Work out the finished part from the listing and answer in its coordinate system (mm). Face numbers are marked on the shaded views. A direction names the side the tool comes from. Give positions to 0.01 mm unless a question says otherwise; leave off trailing zeros. Order: outer loops, then holes, each group sorted by start corner. A loop starts at its lowest first (then second) coordinate and runs counter-clockwise, first axis right, second up.
```python
from build123d import *

# Parameters (mm, degrees)
SKETCH1_R                = 6.5
SKETCH1_R_2              = 5.5
BOSS_EXTRUDE1_DEPTH      = 7.5
BOSS_EXTRUDE2_START      = -2.5
BOSS_EXTRUDE2_DEPTH      = 2.5
M3_CLEARANCE_HOLE1_D     = 3.2
M3_CLEARANCE_HOLE1_DEPTH = 5
M3_CLEARANCE_HOLE1_TIP   = 0.96137699


with BuildPart() as part:
    # Sketch1 → Boss-Extrude1 (new body)
    with BuildSketch(Plane(origin=(0, 0, 0), x_dir=(1, 0, 0), z_dir=(0, 1, 0))):
        with Locations(Location((0, 0, 0), (0, 0, 270))):
            Circle(SKETCH1_R)
        with Locations(Location((0, 0, 0), (0, 0, 270))):
            Circle(SKETCH1_R_2, mode=Mode.SUBTRACT)
    extrude(amount=BOSS_EXTRUDE1_DEPTH)

    # Sketch2 → Boss-Extrude2 (add)
    with BuildSketch(Plane(origin=(0, 7.5, 0), x_dir=(1, 0, 0), z_dir=(0, 1, 0)).offset(BOSS_EXTRUDE2_START)):
        with BuildLine():
            Line((-13.75, 2.5), (-6, 2.5))
            ThreePointArc((-6, 2.5), (-6.5, 0), (-6, -2.5))
            Line((-6, -2.5), (-13.75, -2.5))
            Line((-13.75, -2.5), (-13.75, 2.5))
        make_face()
        with BuildLine():
            Line((13.75, -2.5), (13.75, 2.5))
            Line((13.75, 2.5), (6, 2.5))
            ThreePointArc((6, 2.5), (6.5, 0), (6, -2.5))
            Line((6, -2.5), (13.75, -2.5))
        make_face()
    extrude(amount=BOSS_EXTRUDE2_DEPTH)

    # M3 Clearance Hole1
    with Locations(Plane(origin=(9.875, 5, 0), x_dir=(0, 0, -1), z_dir=(0, -1, 0))):
        with Locations((0, 0), (0, -19.75)):
            Hole(M3_CLEARANCE_HOLE1_D / 2, depth=M3_CLEARANCE_HOLE1_DEPTH)
            with Locations((0, 0, -(M3_CLEARANCE_HOLE1_DEPTH + M3_CLEARANCE_HOLE1_TIP / 2))):  # 118° drill point
                Cone(0, M3_CLEARANCE_HOLE1_D / 2, M3_CLEARANCE_HOLE1_TIP, mode=Mode.SUBTRACT)


solid = part.part
```
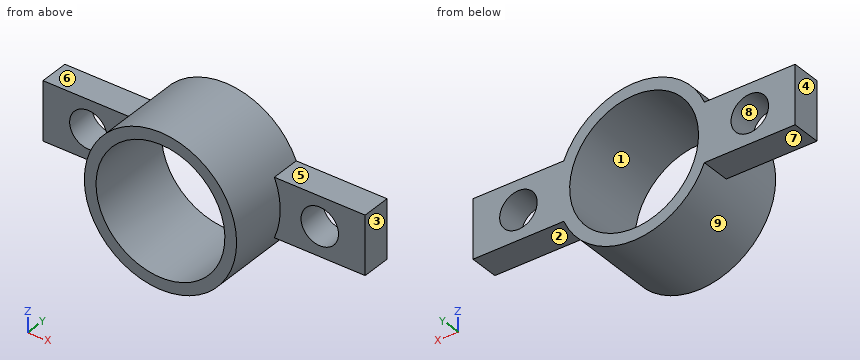
1. The part is cut by section B-B (x = 0). Write down the section's boundary in (y, z), then the cut area to 3 significant figures.
Findings below:
outline: (0, -6.5) - (7.5, -6.5) - (7.5, -5.5) - (0, -5.5) - close; (0, 5.5) - (7.5, 5.5) - (7.5, 6.5) - (0, 6.5) - close
area: 15.0 mm2
2. The part is cut by section A-A (z = 0). Write down the section's boundary in (x, y) (3 decimals).
Findings below:
outline: (-13.75, 5) - (-11.475, 5) - (-11.475, 7.5) - (-13.75, 7.5) - close; (-8.275, 5) - (-6.5, 5) - (-6.5, 0) - (-5.5, 0) - (-5.5, 7.5) - (-8.275, 7.5) - close; (5.5, 0) - (6.5, 0) - (6.5, 5) - (8.275, 5) - (8.275, 7.5) - (5.5, 7.5) - close; (11.475, 5) - (13.75, 5) - (13.75, 7.5) - (11.475, 7.5) - close
3. Which of the six approach directions +Z, -Z, +X, -X, +Y, -Y give full straight-line access (tool end or side, diameter ignored) to the marked faces 5, 6, 7, 8 and 9?
Findings below:
face 5: +Z, +X, +Y, -Y
face 6: +Z, -X, +Y, -Y
face 7: -Z, -X, +Y, -Y
face 8: +Y, -Y
face 9: -Y
4. Given P1, Ø3, axis at x = 10.5, z = 3.5, coming from the -Y side; P2, Ø2, axis at x = -9.5, y = 7, coming from the -Z side; P3, Ø1.5, axis at x = -5.5, z = -5, coming from the +Y side; P4, Ø0.8, axis at x = -8, y = 6.5, coming from the +Z side, each flat-ended and moving along its own axis, determine where each tip first touches the part or whether it passes through.
Findings below:
P1: stops at y = 5
P2: stops at z = -2.5
P3: passes through
P4: stops at z = 2.5
5. The part is cut by section C-C (z = -3). Write down the section's boundary in (x, y).
Findings below:
outline: (-5.77, 0) - (-4.61, 0) - (-4.61, 7.5) - (-5.77, 7.5) - close; (4.61, 0) - (5.77, 0) - (5.77, 7.5) - (4.61, 7.5) - close
6. The part is cut by section D-D (y = 6.5). Write down the section's boundary in (x, z) (3 decimals).
Findings below:
outline: (-13.75, -2.5) - (-6, -2.5) arc R6.5 ccw to (6, -2.5) - (13.75, -2.5) - (13.75, 2.5) - (6, 2.5) arc R6.5 ccw to (-6, 2.5) - (-13.75, 2.5) - close; hole circle Ø3.2 at (-9.875, 0); hole circle Ø11 at (0, 0); hole circle Ø3.2 at (9.875, 0)
7. The mould has two halves that part along X. Classify the marked faces 1, 2, 3 and 4: pulls with the +X half, pulls with the -X half, needs draft (parallel to the pull), parting line crosses it, or undercut.
Findings below:
face 1: undercut
face 2: needs draft
face 3: pulls with the +X half
face 4: pulls with the -X half
8. Straight lines are drawn through the part: probe 1 along X at (y, z) = (5.25, 0) (3 decimals); probe 2 along X at (y, z) = (7, 0.5); probe 3 along Z at (x, y) = (0.25, 5.5). For each, find the intervals that lie inside material, in ascending order.
Findings below:
probe 1: x = -13.75 to -11.475, -8.275 to -5.5, 5.5 to 8.275, 11.475 to 13.75
probe 2: x = -13.75 to -11.39, -8.36 to -5.48, 5.48 to 8.36, 11.39 to 13.75
probe 3: z = -6.5 to -5.49, 5.49 to 6.5
